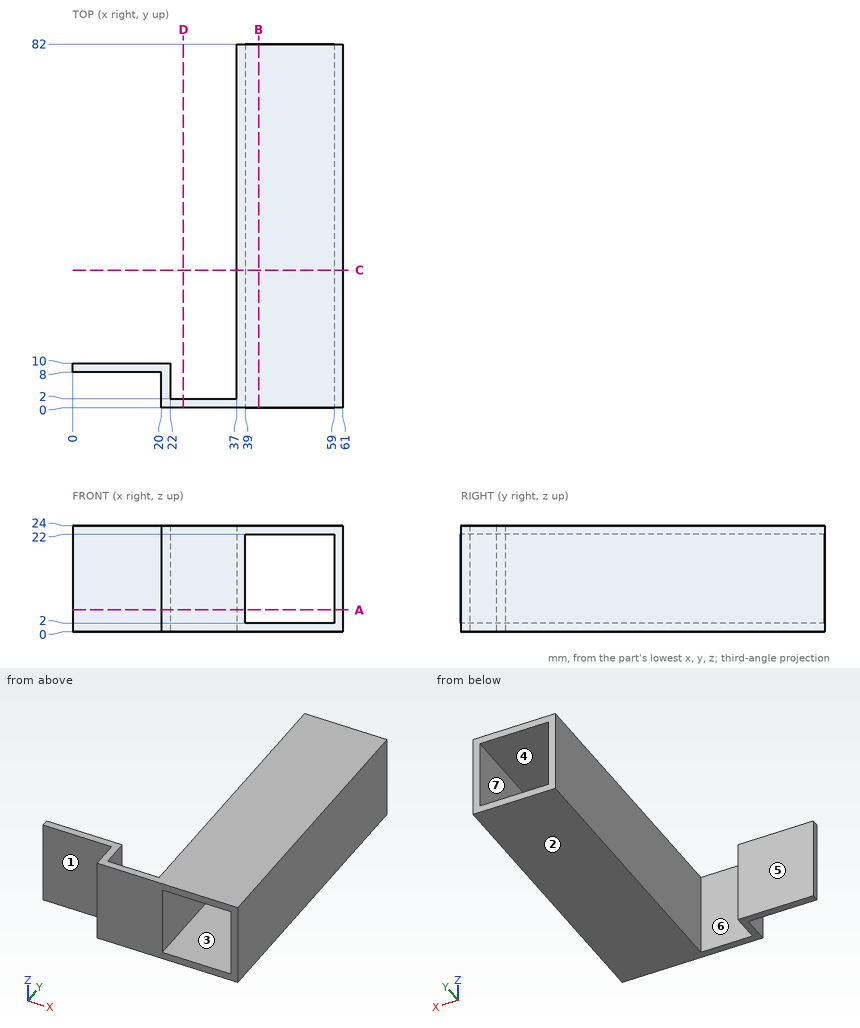
Answer from the drawing. Dimensions are ordinates in mm from the lowest x, y and z of the part. A direction names the side the tool comes from. Round coordinates to 2 decimals unless told otherwise and drop trailing zeros. Loops run counter-clockwise (first coordinate to the right, second up) from the corner with the lowest first, then second, coordinate; pieces in that order, holes last. Notation, with made-up numbers: (21, 71.5) - (61, 71.5) arc R29 ccw to (61, 97.5) - close; hole circle Ø11 at (60.5, -39). An arc over 180 degrees is marked (long way). Return JSON: item names as keys, results as strings. Group by question number.
1. Consider probe 1 along X at (y, z) = (60.5, 12); probe 2 along Z at (x, y) = (47.5, 32); probe 3 along Y at (x, z) = (11, 22). Determine where each line is inside the solid, lowest interval first.
2. The part is cut by section D-D on x = 25. Determine the outline of the cut face in (y, z).
3. Each of these flat-tipped pins is pushed along its axis until it touches: P1, Ø1, axis at y = 63, z = 14, coming from the -X side; P2, Ø1.5, axis at x = 28, z = 5.5, coming from the +Y side; P3, Ø2.5, axis at y = 2.5, z = 12.5, coming from the -X side. Where does it stop, or does it pass through?
4. The part is cut by section A-A on z = 5. Determine the outline of the cut face in (x, y), then the cut area to 3 significant figures.
5. The part is cut by section C-C on y = 31. Determine the outline of the cut face in (x, z), then the cut area to 3 significant figures.
6. The part is cut by section B-B on x = 42. Determine the outline of the cut face in (y, z).
7. Which of the six approach directions +Z, -Z, +X, -X, +Y, -Y give full straight-line access (tool end or side, diameter ignored) to the marked faces 5, 6 and 7?
8. The mould has two halves that part along Z. Classify the marked faces 1, 2, 3 and 4: pulls with the +Z half, pulls with the -Z half, needs draft (parallel to the pull), parting line crosses it, or undercut.
Resolved:
{
 "1": {"probe 1": "x = 37 to 39, 59 to 61", "probe 2": "z = 0 to 2, 22 to 24", "probe 3": "y = 8 to 10"},
 "2": {"outline": "(0, 0) - (2, 0) - (2, 24) - (0, 24) - close"},
 "3": {"P1": "stops at x = 37", "P2": "stops at y = 2", "P3": "stops at x = 20"},
 "4": {"outline": "(0, 8) - (20, 8) - (20, 0) - (39, 0) - (39, 82) - (37, 82) - (37, 2) - (22, 2) - (22, 10) - (0, 10) - close; (59, 0) - (61, 0) - (61, 82) - (59, 82) - close", "area": "418 mm²"},
 "5": {"outline": "(37, 0) - (61, 0) - (61, 24) - (37, 24) - close; hole (39, 2) - (59, 2) - (59, 22) - (39, 22) - close", "area": "176 mm²"},
 "6": {"outline": "(0, 0) - (82, 0) - (82, 2) - (0, 2) - close; (0, 22) - (82, 22) - (82, 24) - (0, 24) - close"},
 "7": {"face 5": "+Z, -Z, -X, +Y", "face 6": "+Z, -Z, +Y", "face 7": "+Y, -Y"},
 "8": {"face 1": "needs draft", "face 2": "pulls with the -Z half", "face 3": "undercut", "face 4": "undercut"}
}
